Design review of the part built by this model. Coordinates are the model's own, in mm. A direction names the side the tool comes from. Give positions to 0.01 mm unless a question says otherwise; leave off trailing zeros. Order: outer loops, then holes, each group sorted by start corner. A loop starts at its lowest first (then second) coordinate and runs counter-clockwise, first axis right, second up. Notation, with made-up numbers: (-32, 58.25) -> (-5, 58.25) arc R19 ccw to (-5, 63.25) -> close; hole circle Ø4 at (16.25, -37.5). An arc over 180 degrees is marked (long way). Return JSON: item names as keys, results as strings.
```python
from build123d import *

# Parameters (mm, degrees)
CHAMFER_1_SIZE = 0.5


with BuildPart() as part:
    # 草图2 → 旋转1 (revolve)
    with BuildSketch(Plane(origin=(0, 0, 0), x_dir=(0, 0, -1), z_dir=(1, 0, 0))):
        Polygon((10, 0), (68.5, 0), (68.5, 6), (38.5, 6), (38.5, 8), (10, 8), align=None)
    revolve(axis=Axis((0, 0, 0), (0, 1, 0)))

    # 倒角1
    chamfer_1_edges = [part.edges().sort_by_distance(p)[0] for p in [
        (0, 0, 68.5),
        (0, 0, 10),
        (0, 8, 10),
        (0, 8, 38.5),
        (0, 6, 68.5),
    ]]
    chamfer(chamfer_1_edges, length=CHAMFER_1_SIZE)


solid = part.part
```
Item 1: Add section A-A (z = 0). Give the boundary of the cut face in (x, y).
Result set:
{"outline": "(-68.5, 0.5) -> (-68, 0) -> (-10.5, 0) -> (-10, 0.5) -> (-10, 7.5) -> (-10.5, 8) -> (-38, 8) -> (-38.5, 7.5) -> (-38.5, 6) -> (-68, 6) -> (-68.5, 5.5) -> close; (10, 0.5) -> (10.5, 0) -> (68, 0) -> (68.5, 0.5) -> (68.5, 5.5) -> (68, 6) -> (38.5, 6) -> (38.5, 7.5) -> (38, 8) -> (10.5, 8) -> (10, 7.5) -> close"}
Item 2: Machinability: for faces 1 (the face through (23.43, 6.76, 30.55)), 2 (the face through (-1, 0, 14)), which of the approach directions +Z, -Z, +X, -X, +Y, -Y give a long, thin tool a straight path to every point of the face, cutting with its end or side? Answer none if there is none.
Result set:
{"face 1": "+Y", "face 2": "+Z, -Z, +X, -X, -Y"}
Item 3: Mouldability with a two-part tool opening along X and no side actions: class faces 3 (the face through (-20.576, 3.035, -65.337)), 4 (the face through (9.76, 3.95, 2.17)), 5 (the face through (29, 6, -29)) as released by +X, released by -X, zero draft, split by the parting line, or undercut.
Result set:
{"face 3": "split by the parting line", "face 4": "undercut", "face 5": "zero draft"}
Item 4: For pin 1 (1 mm diameter, centred on x = 5, y = 2, fed in from +Z); pin 2 (2 mm diameter, centred on y = 1, z = 6, fed in from -X); pin 3 (1 mm diameter, centred on x = -9.5, z = 41, fed in from +Y); pin 4 (12 mm diameter, centred on x = 0, z = 0, fed in from +Y), all flat-tipped, find the tip position at first contact; note any pin that passes through.
Result set:
{"pin 1": "stops at z = 68.35", "pin 2": "stops at x = -68.32", "pin 3": "stops at y = 6", "pin 4": "passes through"}
Item 5: Add section B-B (x = 0). Give the boundary of the cut face in (y, z), plus the area to 3 significant figures.
Result set:
{"outline": "(0, -68) -> (0.5, -68.5) -> (5.5, -68.5) -> (6, -68) -> (6, -38.5) -> (7.5, -38.5) -> (8, -38) -> (8, -10.5) -> (7.5, -10) -> (0.5, -10) -> (0, -10.5) -> close; (0, 10.5) -> (0.5, 10) -> (7.5, 10) -> (8, 10.5) -> (8, 38) -> (7.5, 38.5) -> (6, 38.5) -> (6, 68) -> (5.5, 68.5) -> (0.5, 68.5) -> (0, 68) -> close", "area": "815 mm^2"}
Item 6: Wall thickness on L1, parallel to Z at x = 0, y = 4.5; L2, parallel to Y at x = 6.5, z = -46: over which ranges is each line inside the solid? List them lowest first. Write a range as [from, to].
Result set:
{"L1": "z = [-68.5, -10], [10, 68.5]", "L2": "y = [0, 6]"}
Item 7: Add section C-C (y = 2.5). Give the boundary of the cut face in (x, z).
Result set:
{"outline": "circle Ø137 at (0, 0); hole circle Ø20 at (0, 0)"}
